Could you check a few things on this model? Use its own coordinates, in mm. A direction names the side the tool comes from. Round coordinates to 2 decimals unless told otherwise and drop trailing zeros. Order: outer loops, then holes, each group sorted by start corner. A loop starts at its lowest first (then second) coordinate and runs counter-clockwise, first axis right, second up.
Autodesk Inventor part; units mm, degrees
ref_plane "YZ Plane" through (0, 0, 0) normal (1, 0, 0) x (0, 1, 0)
ref_plane "XZ Plane" through (0, 0, 0) normal (0, 1, 0) x (-1, 0, 0)
ref_plane "XY Plane" through (0, 0, 0) normal (0, 0, 1) x (1, 0, 0)
sketch "Boceto1" plane through (0, 0, 0) normal (0, 1, 0) x (-1, 0, 0)
  circle A0 centre (0, 0) radius 22
  dimension "d0" = 44
extrude "Extrusión1" add sketch "Boceto1" along normal blind 20
shell "Vaciado1" thickness 1 removed faces 1 at (6.4933, 20, -3.408)
sketch "Boceto3" plane through (0, 1, 0) normal (0, 1, 0) x (1, 0, 0)
  circle A0 centre (0, 0) radius 21
  line L0 (2.4, 19.75) -> (-2.4, 19.75)
  line L1 (-2.4, 19.75) -> (-2.4, 22.25)
  line L2 (-2.4, 22.25) -> (2.4, 22.25)
  line L3 (2.4, 22.25) -> (2.4, 19.75)
  line L4 (2.4, 19.75) -> (-2.4, 22.25) construction
  line L5 (-2.4, 19.75) -> (2.4, 22.25) construction
  point P0 (0, 21)
  dimension "d4" = 4.8
  dimension "d5" = 2.5
extrude "Extrusión2" cut sketch "Boceto3" along normal blind 2.5 contours L3 L0 L1 A0 | A0 L1 L2 L3 picked at (-0.2672, 20.1616)
fillet "Empalme1" radius 2 2 edges at (22, 0, 0) (21, 20, 0)
properties part number "Tapa motor775"
Q1. For P1, Ø5, axis at x = -17.5, y = 9.5, coming from the -Z side; P2, Ø3, axis at y = 7, z = 13, coming from the +X side (3 decimals); P3, Ø12, axis at x = -3, y = 15.5, coming from the +Z side; P4, Ø12, axis at x = -1, y = 13.5, coming from the -Z side, each with a flat end and sliding along its axis, tell me the tip position at first contact or that it passes through.
Q2. For faces 4 (the cylindrical face through (-20.03, 9.51, -6.31)), 5 (the flat face through (0, 3.5, -21.4)), which set-ups out of +Z, -Z, +X, -X, +Y, -Y let a thin tool reach every point of the face, with its end or its side?
Q3. I need wall thicknesses on L1, parallel to X at y = 5.75, z = 0; L2, parallel to Y at x = 1.5, z = 3.5. Which ranges of each line are inside material? Lowest first, please.
Q4. Imagine slicing it at A-A, the plane x = 0. Please give me the cut outline in (y, z).
Q5. Imagine slicing it at B-B, the plane z = 0. Please give me the cut outline in (x, y).
Q6. We'd pull the mould along X, two halves only. Please class faces 1 (the flat face through (0, 0, 0)), 2 (the flat face through (0, 1, -1)), 3 (the cylindrical face through (4.769, 10.874, 21.477)): released by +X, released by -X, zero draft, split by the parting line, or undercut.
Filled in:
1. P1: stops at z = -16.09
1. P2: stops at x = 18.755
1. P3: stops at z = 22
1. P4: stops at z = -22
2. face 4: +Y
2. face 5: -Z
3. L1: x = -22 to -21, 21 to 22
3. L2: y = 0 to 1
4. outline: (0, -20) arc R2 ccw to (1, -21.73) - (1, 21) - (18.27, 21) arc R2 ccw to (20, 22) - (2, 22) arc R2 ccw to (0, 20) - close; (3.5, -22) - (20, -22) arc R2 ccw to (18.27, -21) - (3.5, -21) - close
5. outline: (-22, 2) arc R2 ccw to (-20, 0) - (20, 0) arc R2 ccw to (22, 2) - (22, 20) arc R2 ccw to (21, 18.27) - (21, 1) - (-21, 1) - (-21, 18.27) arc R2 ccw to (-22, 20) - close
6. face 1: zero draft
6. face 2: undercut
6. face 3: split by the parting line
